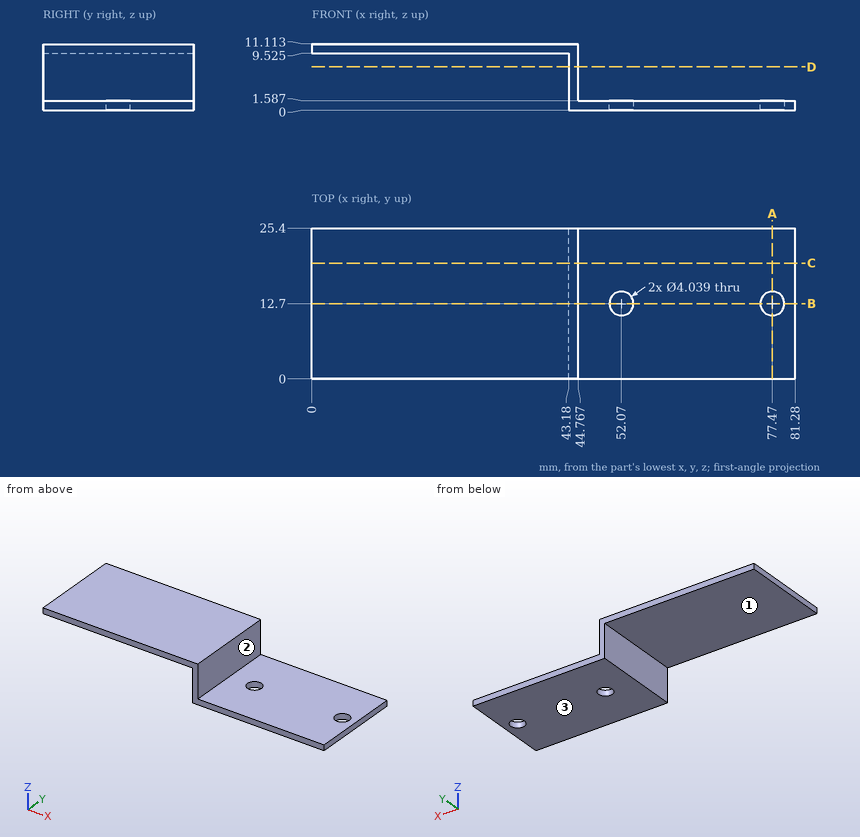
Geometry check sheet. Reference: drawing and pictorial views, mm from the part's lowest x, y, z. A direction names the side the tool comes from. Coordinates: 2 decimals unless noted, no trailing zeros. Loops run counter-clockwise (first coordinate to the right, second up) from the corner with the lowest first, then second, coordinate; pieces in that order, holes last. Notation, with made-up numbers: (46.5, 12) -> (53.5, 12) arc R20 ccw to (53.5, 42) -> close; hole circle Ø2 at (9, -22.75). An arc over 180 degrees is marked (long way). Write item = value, one per line. Start each with the question number.
1. Section check C-C on y = 19.5. Record the cut outline in (x, z) (1 decimal).
2. Tool access check on the marked faces 1, 2 and 3. Record the directions out of +Z, -Z, +X, -X, +Y, -Y that give a thin tool (end or side, any length) a straight path to the whole face; none if there is none.
3. Section check B-B on y = 12.7. Give the number of separate pieces and of enclosed holes in the cut face.
4. Section check D-D on z = 7.25. Record the cut outline in (x, y).
5. Section check A-A on x = 77.47. Record the cut outline in (y, z).
6. Depth check by flat-ended pin: P1, Ø3, axis at y = 11, z = 5.5, coming from the +X side; P2, Ø12.5, axis at x = 72, y = 7.5, coming from the +Z side; P3, Ø2, axis at y = 17, z = 2, coming from the -X side; P4, Ø3, axis at x = 52.07, y = 12.7, coming from the +Z side (3 decimals). Enter the tip coordinate at first touch or a pass-through.
7. Material ranges on line 1 (Y direction, x = 52.07, z = 1.25); line 2 (Z direction, x = 12.5, y = 4.5) (1 decimal); line 3 (Z direction, x = 48, y = 11), recorded low to high.
Responses:
q1.outline = (0, 9.5) -> (43.2, 9.5) -> (43.2, 0) -> (81.3, 0) -> (81.3, 1.6) -> (44.8, 1.6) -> (44.8, 11.1) -> (0, 11.1) -> close
q2.face_1 = -Z, -X, +Y, -Y
q2.face_2 = +Z, +X, +Y, -Y
q2.face_3 = -Z, +X, -X, +Y, -Y
q3.separate_pieces = 3
q3.enclosed_holes = 0
q4.outline = (43.18, 0) -> (44.77, 0) -> (44.77, 25.4) -> (43.18, 25.4) -> close
q5.outline = (0, 0) -> (10.68, 0) -> (10.68, 1.59) -> (0, 1.59) -> close; (14.72, 0) -> (25.4, 0) -> (25.4, 1.59) -> (14.72, 1.59) -> close
q6.P1 = 44.77
q6.P2 = 1.59
q6.P3 = 43.18
q6.P4 = through
q7.line_1 = 0 to 10.68, 14.72 to 25.4
q7.line_2 = 9.5 to 11.1
q7.line_3 = 0 to 1.59
